Could you check a few things on this model? Use its own coordinates, in mm. A direction names the side the tool comes from. Give positions to 0.01 mm unless a question says otherwise; leave off trailing zeros. Order: outer loops, then holes, each group sorted by start corner. A loop starts at its lowest first (then second) coordinate and runs counter-clockwise, first axis right, second up.
from build123d import *

# Parameters (mm, degrees)
SKETCH1_W           = 30
SKETCH1_H           = 30
BOSS_EXTRUDE1_DEPTH = 4
SKETCH2_W           = 5
SKETCH2_H           = 30
BOSS_EXTRUDE2_DEPTH = 30
SKETCH3_W           = 30
SKETCH3_H           = 4
BOSS_EXTRUDE3_DEPTH = 28
SKETCH4_W           = 4
SKETCH4_H           = 30
BOSS_EXTRUDE4_DEPTH = 6
FILLET1_R           = 1


with BuildPart() as part:
    # Sketch1 → Boss-Extrude1 (new body)
    with BuildSketch(Plane(origin=(0, 0, 0), x_dir=(1, 0, 0), z_dir=(0, 1, 0))):
        with Locations((15, 15)):
            Rectangle(SKETCH1_W, SKETCH1_H)
    extrude(amount=BOSS_EXTRUDE1_DEPTH)

    # Sketch2 → Boss-Extrude2 (add)
    with BuildSketch(Plane(origin=(0, 4, 0), x_dir=(1, 0, 0), z_dir=(0, 1, 0))):
        with Locations((27.5, 15)):
            Rectangle(SKETCH2_W, SKETCH2_H)
    extrude(amount=BOSS_EXTRUDE2_DEPTH)

    # Sketch3 → Boss-Extrude3 (add)
    with BuildSketch(Plane.ZY.offset(-25)):
        with Locations((-15, 32)):
            Rectangle(SKETCH3_W, SKETCH3_H)
    extrude(amount=BOSS_EXTRUDE3_DEPTH)

    # Sketch4 → Boss-Extrude4 (add)
    with BuildSketch(Plane.XZ.offset(-30)):
        with Locations((-1, -15)):
            Rectangle(SKETCH4_W, SKETCH4_H)
    extrude(amount=BOSS_EXTRUDE4_DEPTH)

    # Fillet1
    fillet1_edges = [part.edges().sort_by_distance(p)[0] for p in [
        (0, 4, -15),
        (30, 34, -15),
        (-3, 34, -15),
    ]]
    fillet(fillet1_edges, radius=FILLET1_R)


solid = part.part
Item 1: Please list where these lines run through material, in increasing order: line 1 along X through (y, z) = (29, -16); line 2 along Y through (x, z) = (2.5, -1.25); line 3 along X through (y, z) = (9, -28.25).
Findings:
line 1: x = -3 to 1, 25 to 30
line 2: y = 0 to 4, 30 to 34
line 3: x = 25 to 30
Item 2: For pin 1 (13 mm diameter, centred on y = 17, z = -8.5, fed in from -X); pin 2 (0.9 mm diameter, centred on y = 1, z = -21, fed in from -X), each with a flat end and sliding along its axis, tell me the tip position at first contact or that it passes through.
Findings:
pin 1: stops at x = 25
pin 2: stops at x = 0
Item 3: Imagine slicing it at D-D on y = 6. List the corners of the cut face in (x, z) for me.
Findings:
outline: (25, -30) - (30, -30) - (30, 0) - (25, 0) - close
Item 4: Imagine slicing it at A-A on x = 2. List the corners of the cut face in (y, z) for me, then the cut area to 3 significant figures.
Findings:
outline: (0, -30) - (4, -30) - (4, 0) - (0, 0) - close; (30, -30) - (34, -30) - (34, 0) - (30, 0) - close
area: 240 mm2
Item 5: Imagine slicing it at B-B on y = 24.5. List the corners of the cut face in (x, z) for me, then the cut area to 3 significant figures.
Findings:
outline: (-3, -30) - (1, -30) - (1, 0) - (-3, 0) - close; (25, -30) - (30, -30) - (30, 0) - (25, 0) - close
area: 270 mm2
Item 6: We'd pull the mould along Y, two halves only. Please class faces 1 (the cylindrical face through (-2.715, 33.699, -14.79)), 2 (the flat face through (-1, 24, -15)), 3 (the flat face through (26, 17, -30)): +Y half, -Y half, draft (parallel to the pull), parting line (faces both ways), or undercut.
Findings:
face 1: +Y half
face 2: undercut
face 3: draft
Item 7: Imagine slicing it at C-C on z = -16. List the corners of the cut face in (x, y) for me, then the cut area to 3 significant figures.
Findings:
outline: (-3, 24) - (1, 24) - (1, 30) - (25, 30) - (25, 4) - (1, 4) arc R1 ccw to (0, 3) - (0, 0) - (30, 0) - (30, 33) arc R1 ccw to (29, 34) - (-2, 34) arc R1 ccw to (-3, 33) - close
area: 405 mm2
Item 8: For faces 4 (the cylindrical face through (0.285, 3.699, -15.21)), 5 (the flat face through (1, 27, -15)), 6 (the flat face through (30, 16, -15)), 7 (the flat face through (0, 1, -15)), which set-ups out of +Z, -Z, +X, -X, +Y, -Y let a thin tool reach every point of the face, with its end or its side?
Findings:
face 4: +Z, -Z, -X
face 5: +Z, -Z
face 6: +Z, -Z, +X, +Y, -Y
face 7: +Z, -Z, -X, -Y
